```python
from build123d import *

# Parameters (mm, degrees)
SKETCH_1_W             = 110
SKETCH_1_H             = 58
SM_BASE_FLANGE_1_DEPTH = 3.6
CUT_EXTRUDE_1_REACH    = 126.406
SKETCH_2_W             = 3.6
SKETCH_2_H             = 16
SKETCH_3_W             = 22
SKETCH_3_H             = 3.6
EXTRUDE_1_DEPTH        = 3.6


# Sheet-metal steps are written as plain solids
with BuildPart() as part:
    # Sketch 1 → Базовая кромка1 (new body)
    with BuildSketch(Plane.XY):
        with Locations((55, 29)):
            Rectangle(SKETCH_1_W, SKETCH_1_H)
    extrude(amount=-SM_BASE_FLANGE_1_DEPTH)

    # Sketch 2 → Вырез-Вытянуть1 (cut, up to next)
    with BuildSketch(Plane(origin=(0, 0, -3.6), x_dir=(-1, 0, 0), z_dir=(0, 0, -1)), mode=Mode.PRIVATE) as cut_extrude_1_sk1:
        with Locations((-108.2, 42)):
            Rectangle(SKETCH_2_W, SKETCH_2_H)
    cut_extrude_1_tool1 = extrude(cut_extrude_1_sk1.sketch, amount=-CUT_EXTRUDE_1_REACH, mode=Mode.PRIVATE) & part.part
    # Sketch 2 → Вырез-Вытянуть1 (cut, up to next)
    with BuildSketch(Plane(origin=(0, 0, -3.6), x_dir=(-1, 0, 0), z_dir=(0, 0, -1)), mode=Mode.PRIVATE) as cut_extrude_1_sk2:
        with Locations((-108.2, 16)):
            Rectangle(SKETCH_2_W, SKETCH_2_H)
    cut_extrude_1_tool2 = extrude(cut_extrude_1_sk2.sketch, amount=-CUT_EXTRUDE_1_REACH, mode=Mode.PRIVATE) & part.part
    # Sketch 2 → Вырез-Вытянуть1 (cut, up to next)
    with BuildSketch(Plane(origin=(0, 0, -3.6), x_dir=(-1, 0, 0), z_dir=(0, 0, -1)), mode=Mode.PRIVATE) as cut_extrude_1_sk3:
        with Locations((-1.8, 16)):
            Rectangle(SKETCH_2_W, SKETCH_2_H)
    cut_extrude_1_tool3 = extrude(cut_extrude_1_sk3.sketch, amount=-CUT_EXTRUDE_1_REACH, mode=Mode.PRIVATE) & part.part
    # Sketch 2 → Вырез-Вытянуть1 (cut, up to next)
    with BuildSketch(Plane(origin=(0, 0, -3.6), x_dir=(-1, 0, 0), z_dir=(0, 0, -1)), mode=Mode.PRIVATE) as cut_extrude_1_sk4:
        with Locations((-1.8, 42)):
            Rectangle(SKETCH_2_W, SKETCH_2_H)
    cut_extrude_1_tool4 = extrude(cut_extrude_1_sk4.sketch, amount=-CUT_EXTRUDE_1_REACH, mode=Mode.PRIVATE) & part.part
    add(cut_extrude_1_tool1.solids().sort_by_distance((108.2, 42, -3.6))[0], mode=Mode.SUBTRACT)
    add(cut_extrude_1_tool2.solids().sort_by_distance((108.2, 16, -3.6))[0], mode=Mode.SUBTRACT)
    add(cut_extrude_1_tool3.solids().sort_by_distance((1.8, 16, -3.6))[0], mode=Mode.SUBTRACT)
    add(cut_extrude_1_tool4.solids().sort_by_distance((1.8, 42, -3.6))[0], mode=Mode.SUBTRACT)

    # Эскиз3 → Бобышка-Вытянуть1 (add)
    with BuildSketch(Plane.XY):
        with Locations((23, 59.8)):
            Rectangle(SKETCH_3_W, SKETCH_3_H)
        with Locations((87, 59.8)):
            Rectangle(SKETCH_3_W, SKETCH_3_H)
        with Locations((23, -1.8)):
            Rectangle(SKETCH_3_W, SKETCH_3_H)
        with Locations((87, -1.8)):
            Rectangle(SKETCH_3_W, SKETCH_3_H)
    extrude(amount=-EXTRUDE_1_DEPTH)


solid = part.part
```
For this review, take the finished solid that the model builds, in its own axes (mm). A direction names the side the tool comes from. Coordinates: 2 decimals unless noted, no trailing zeros. Order: outer loops, then holes, each group sorted by start corner. A loop starts at its lowest first (then second) coordinate and runs counter-clockwise, first axis right, second up. Notation, with made-up numbers: (63.25, 48) -> (113.25, 48) arc R13 ccw to (113.25, 62) -> close; hole circle Ø11 at (25.25, 64.25). An arc over 180 degrees is marked (long way). Use CSV: the item, a comma, the result in double quotes. Start each with the question number.
Item 1: Draft analysis for pull direction X (two halves, no side actions). For faces 6 (the face through (55, 0, -2)), 7 (the face through (12, 60, -2)), 8 (the face through (54, 29, 0)), state which applies: pulls with the +X half, pulls with the -X half, needs draft (parallel to the pull), parting line crosses it, or undercut.
Item 2: Insertion check: pin 1 (1.8 mm diameter, centred on x = 109, z = -1, fed in from +Y); pin 2 (1.1 mm diameter, centred on y = 16.5, z = -2, fed in from +X); pin 3 (1.1 mm diameter, centred on y = 60.5, z = -2.5, fed in from -X). Each pin has a flat end and moves straight along its axis. Give the tip position at first contact, or say it passes through.
Item 3: Wall thickness on probe 1 along X at (y, z) = (40.5, -1.75); probe 2 along Y at (x, z) = (66.5, -0.75): over which ranges is each line inside the solid? List them lowest first.
Item 4: For faces 1 (the face through (3.6, 42, -2)), 2 (the face through (108, 8, -2)), 3 (the face through (104, 58, -2)), 4 (the face through (110, 4, -2)), 5 (the face through (34, -2, -2)), list the 3-axis set-ups (+Z, -Z, +X, -X, +Y, -Y) from which the entire face can be reached by the end or side of a thin tool; tool diameter is ignored.
Item 5: We need section B-B, the plane y = 40.5. Give the boundary of the cut face in (x, z), then the cut area to 3 significant figures.
Item 6: We need section A-A, the plane x = 9.5. Give the boundary of the cut face in (y, z).
Derived:
1,face 6,"undercut"
1,face 7,"pulls with the -X half"
1,face 8,"needs draft"
2,pin 1,"stops at y = 58"
2,pin 2,"stops at x = 106.4"
2,pin 3,"stops at x = 12"
3,probe 1,"x = 3.6 to 106.4"
3,probe 2,"y = 0 to 58"
4,face 1,"+Z, -Z, -X"
4,face 2,"+Z, -Z, +X"
4,face 3,"+Z, -Z, +X, +Y"
4,face 4,"+Z, -Z, +X, +Y, -Y"
4,face 5,"+Z, -Z, -Y"
5,outline,"(3.6, -3.6) -> (106.4, -3.6) -> (106.4, 0) -> (3.6, 0) -> close"
5,area,"370 mm^2"
6,outline,"(0, -3.6) -> (58, -3.6) -> (58, 0) -> (0, 0) -> close"
